from build123d import *

# Parameters (mm, degrees)
SKETCH1_W           = 133.5
SKETCH1_H           = 126.4
SKETCH1_R           = 2.6
SKETCH1_R_2         = 1.6
SKETCH1_W_2         = 5
SKETCH1_H_2         = 10
BOSS_EXTRUDE1_DEPTH = 5
CUT_EXTRUDE2_DEPTH  = 10
FILLET2_R           = 10
CUT_EXTRUDE3_REACH  = 94.059
SKETCH5_R           = 1.6
SKETCH5_R_2         = 1.5
FILLET3_R           = 1


with BuildPart() as part:
    # Sketch1 → Boss-Extrude1 (new body)
    with BuildSketch(Plane(origin=(0, 0, 0), x_dir=(1, 0, 0), z_dir=(0, 1, 0))):
        Rectangle(SKETCH1_W, SKETCH1_H)
        with Locations(Location((-59.75, -35.7, 0), (0, 0, 270))):
            Circle(SKETCH1_R, mode=Mode.SUBTRACT)
        with Locations(Location((59.75, -35.7, 0), (0, 0, 90))):
            Circle(SKETCH1_R, mode=Mode.SUBTRACT)
        with Locations(Location((-48.05, -48.2, 0), (0, 0, 270))):
            Circle(SKETCH1_R_2, mode=Mode.SUBTRACT)
        with Locations(Location((48.05, -48.2, 0), (0, 0, 90))):
            Circle(SKETCH1_R_2, mode=Mode.SUBTRACT)
        with Locations(Location((-59.75, -10.7, 0), (0, 0, 90))):
            Circle(SKETCH1_R, mode=Mode.SUBTRACT)
        with Locations(Location((59.75, -10.7, 0), (0, 0, 270))):
            Circle(SKETCH1_R, mode=Mode.SUBTRACT)
        with Locations((-59.75, -48.2)):
            Rectangle(SKETCH1_W_2, SKETCH1_H_2, mode=Mode.SUBTRACT)
        with Locations((-59.75, -23.2)):
            Rectangle(SKETCH1_W_2, SKETCH1_H_2, mode=Mode.SUBTRACT)
        with Locations((59.75, -23.2)):
            Rectangle(SKETCH1_W_2, SKETCH1_H_2, mode=Mode.SUBTRACT)
        with Locations((59.75, -48.2)):
            Rectangle(SKETCH1_W_2, SKETCH1_H_2, mode=Mode.SUBTRACT)
        with Locations((-59.75, 1.8)):
            Rectangle(SKETCH1_W_2, SKETCH1_H_2, mode=Mode.SUBTRACT)
        with Locations((59.75, 1.8)):
            Rectangle(SKETCH1_W_2, SKETCH1_H_2, mode=Mode.SUBTRACT)
    extrude(amount=BOSS_EXTRUDE1_DEPTH)

    # Sketch2 → Cut-Extrude2 (cut)
    with BuildSketch(Plane(origin=(0, 5, 0), x_dir=(1, 0, 0), z_dir=(0, 1, 0))):
        with BuildLine():
            Line((-28.75, 86.678700037), (-28.75, 0))
            ThreePointArc((-28.75, 0), (0, -28.75), (28.75, 0))
            Line((28.75, 0), (28.75, 86.678700037))
            Line((28.75, 86.678700037), (-28.75, 86.678700037))
        make_face()
    extrude(amount=-CUT_EXTRUDE2_DEPTH, mode=Mode.SUBTRACT)

    # Fillet2
    fillet2_edges = [part.edges().sort_by_distance(p)[0] for p in [
        (-28.75, 2.5, -63.2),
        (28.75, 2.5, -63.2),
        (-66.75, 2.5, -63.2),
        (66.75, 2.5, -63.2),
    ]]
    fillet(fillet2_edges, radius=FILLET2_R)

    # Sketch5 → Cut-Extrude3 (cut, up to next)
    with BuildSketch(Plane.XZ, mode=Mode.PRIVATE) as cut_extrude3_sk1:
        with Locations(Location((48.05, 23.2, 0), (0, 0, 270))):
            Circle(SKETCH5_R)
    cut_extrude3_tool1 = extrude(cut_extrude3_sk1.sketch, amount=-CUT_EXTRUDE3_REACH, mode=Mode.PRIVATE) & part.part
    # Sketch5 → Cut-Extrude3 (cut, up to next)
    with BuildSketch(Plane.XZ, mode=Mode.PRIVATE) as cut_extrude3_sk2:
        with Locations(Location((48.05, -53.2, 0), (0, 0, 270))):
            Circle(SKETCH5_R_2)
    cut_extrude3_tool2 = extrude(cut_extrude3_sk2.sketch, amount=-CUT_EXTRUDE3_REACH, mode=Mode.PRIVATE) & part.part
    # Sketch5 → Cut-Extrude3 (cut, up to next)
    with BuildSketch(Plane.XZ, mode=Mode.PRIVATE) as cut_extrude3_sk3:
        with Locations(Location((-48.05, -53.2, 0), (0, 0, 90))):
            Circle(SKETCH5_R_2)
    cut_extrude3_tool3 = extrude(cut_extrude3_sk3.sketch, amount=-CUT_EXTRUDE3_REACH, mode=Mode.PRIVATE) & part.part
    # Sketch5 → Cut-Extrude3 (cut, up to next)
    with BuildSketch(Plane.XZ, mode=Mode.PRIVATE) as cut_extrude3_sk4:
        with Locations(Location((-48.05, 23.2, 0), (0, 0, 90))):
            Circle(SKETCH5_R)
    cut_extrude3_tool4 = extrude(cut_extrude3_sk4.sketch, amount=-CUT_EXTRUDE3_REACH, mode=Mode.PRIVATE) & part.part
    add(cut_extrude3_tool1.solids().sort_by_distance((48.05, 0, 23.2))[0], mode=Mode.SUBTRACT)
    add(cut_extrude3_tool2.solids().sort_by_distance((48.05, 0, -53.2))[0], mode=Mode.SUBTRACT)
    add(cut_extrude3_tool3.solids().sort_by_distance((-48.05, 0, -53.2))[0], mode=Mode.SUBTRACT)
    add(cut_extrude3_tool4.solids().sort_by_distance((-48.05, 0, 23.2))[0], mode=Mode.SUBTRACT)

    # Fillet3
    fillet3_edges = [part.edges().sort_by_distance(p)[0] for p in [
        (66.75, 2.5, 63.2),
        (-66.75, 2.5, 63.2),
    ]]
    fillet(fillet3_edges, radius=FILLET3_R)


solid = part.part
Could you check a few things on this model? Use its own coordinates, in mm. A direction names the side the tool comes from. Give positions to 0.01 mm unless a question says otherwise; leave off trailing zeros. Loops run counter-clockwise (first coordinate to the right, second up) from the corner with the lowest first, then second, coordinate; pieces in that order, holes last. Notation, with made-up numbers: (53.5, -11) -> (107.5, -11) arc R13 cw to (107.5, 8) -> close; hole circle Ø4 at (82.5, 57). An arc over 180 degrees is marked (long way). Answer as CSV lines item,"result". Start each with the question number.
(1) I need wall thicknesses on probe 1 along X at (y, z) = (1.8, 24.5); probe 2 along X at (y, z) = (3.5, 20); probe 3 along X at (y, z) = (2.4, -15.5). Which ranges of each line are inside material? Lowest first, please.
(2) Which directions (+Z, -Z, +X, -X, +Y, -Y) give clear straight access to the entire face, cutting with the end or side of a thin tool? Please do faces 4 (the flat face through (-48, 2, -63.2)), 5 (the cylindrical face through (31.6, 2.46, -60.19)), 6 (the flat face through (57.25, 2, 48)).
(3) If we section it at C-C on x = -48.05: Write out the boundary of the cut face in (y, z), then the cut area to 3 significant figures.
(4) I'm going to push flat-ended pins straight in: pin 1 Ø1.9 at (x, z) = (48.05, 48.2) entering from -Y; pin 2 Ø1 at (x, y) = (-13, 3) entering from -Z; pin 3 Ø2.5 at (x, y) = (59, 2) entering from -Z. Where does each tip first touch, or does it pass through?
(5) If we section it at B-B on z = 35.7: Write out the boundary of the cut face in (x, y), then the cut area to 4 significant figures.
(6) If we section it at D-D on x = 59.75: Write out the boundary of the cut face in (y, z), then the cut area to 3 significant figures.
(7) We'd pull the mould along X, two halves only. Please class faces 1 (the flat face through (-1, 2, 63.2)), 2 (the flat face through (66.75, 2, 5)), 3 (the flat face through (-60, 2, 43.2)): released by +X, released by -X, zero draft, split by the parting line, or undercut.
(8) If we section it at A-A on z = -35: Write out the boundary of the cut face in (x, y), then the cut area to 3 significant figures.
Computed:
1,probe 1,"x = -66.75 to -62.25, -57.25 to -48.98, -47.12 to -15.04, 15.04 to 47.12, 48.98 to 57.25, 62.25 to 66.75"
1,probe 2,"x = -66.75 to -62.25, -57.25 to -20.65, 20.65 to 57.25, 62.25 to 66.75"
1,probe 3,"x = -66.75 to -28.75, 28.75 to 66.75"
2,face 4,"-Z, +X, -X, +Y, -Y"
2,face 5,"-Z, +Y, -Y"
2,face 6,"+Y, -Y"
3,outline,"(0, -63.2) -> (5, -63.2) -> (5, -54.7) -> (0, -54.7) -> close; (0, -51.7) -> (5, -51.7) -> (5, 21.6) -> (0, 21.6) -> close; (0, 24.8) -> (5, 24.8) -> (5, 46.6) -> (0, 46.6) -> close; (0, 49.8) -> (5, 49.8) -> (5, 63.2) -> (0, 63.2) -> close"
3,area,"585 mm2"
4,pin 1,"passes through"
4,pin 2,"stops at z = 25.38"
4,pin 3,"stops at z = -63.15"
5,outline,"(-66.75, 0) -> (-62.35, 0) -> (-62.35, 5) -> (-66.75, 5) -> close; (-57.15, 0) -> (57.15, 0) -> (57.15, 5) -> (-57.15, 5) -> close; (62.35, 0) -> (66.75, 0) -> (66.75, 5) -> (62.35, 5) -> close"
5,area,"615.5 mm2"
6,outline,"(0, -62.74) -> (5, -62.74) -> (5, -6.8) -> (0, -6.8) -> close; (0, 3.2) -> (5, 3.2) -> (5, 8.1) -> (0, 8.1) -> close; (0, 13.3) -> (5, 13.3) -> (5, 18.2) -> (0, 18.2) -> close; (0, 28.2) -> (5, 28.2) -> (5, 33.1) -> (0, 33.1) -> close; (0, 38.3) -> (5, 38.3) -> (5, 43.2) -> (0, 43.2) -> close; (0, 53.2) -> (5, 53.2) -> (5, 63.2) -> (0, 63.2) -> close"
6,area,"428 mm2"
7,face 1,"zero draft"
7,face 2,"released by +X"
7,face 3,"undercut"
8,outline,"(-66.75, 0) -> (-28.75, 0) -> (-28.75, 5) -> (-66.75, 5) -> close; (28.75, 0) -> (66.75, 0) -> (66.75, 5) -> (28.75, 5) -> close"
8,area,"380 mm2"
